Answer from the drawing. Dimensions are ordinates in mm from the lowest x, y and z of the part. A direction names the side the tool comes from. Coordinates: 2 decimals unless noted, no trailing zeros. Write each loop counter-clockwise with the first axis right and the second up, starting at its lowest first coordinate (ties: lowest second). Pieces come first, ordered by that corner, then holes.
(1) Given pin 1 (2 mm diameter, centred on y = 29.5, z = 9, fed in from +X); pin 2 (6 mm diameter, centred on x = 9, y = 26, fed in from -Z), each flat-ended and moving along its own axis, determine where each tip first touches the part or whether it passes through.
(2) Section D-D on y = 10 is taken. Write down the section's boundary in (x, z), then the cut area to 3 significant figures.
(3) Section A-A on z = 3.5 is taken. Write down the section's boundary in (x, y).
(4) The mould has two halves that part along Y. Classify the marked faces 1, 2 and 3: +Y half, -Y half, draft (parallel to the pull), parting line (faces both ways), or undercut.
(5) Find the intervals of material crossed by probe 1 along Y at (x, z) = (3.5, 9.5); probe 2 along Y at (x, z) = (6.5, 1); probe 3 along Z at (x, y) = (5.25, 4), in increasing order.
(6) Section C-C on x = 1 is taken. Write down the section's boundary in (y, z).
(7) Section B-B on y = 32 is taken. Write down the section's boundary in (x, z).
(8) Which of the six approach directions +Z, -Z, +X, -X, +Y, -Y give full straight-line access (tool end or side, diameter ignored) to the marked faces 4, 5 and 6?
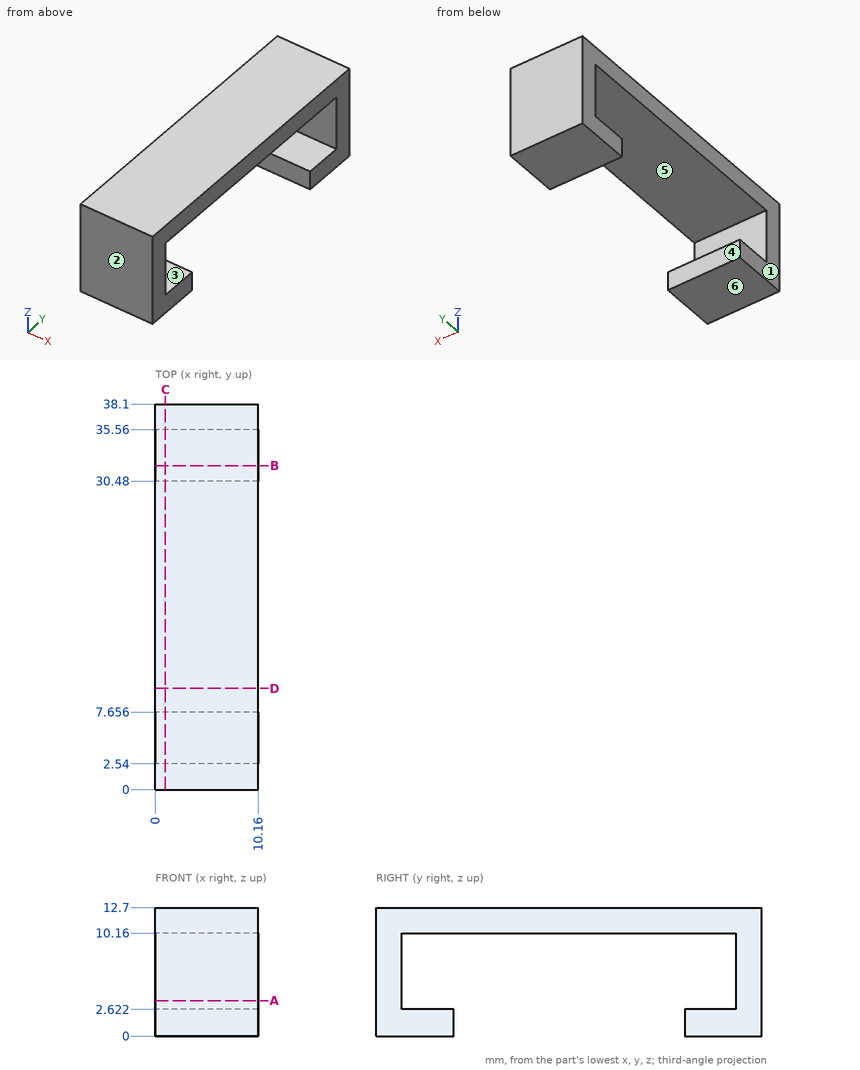
Response:
1. pin 1: passes through
1. pin 2: stops at z = 10.16
2. outline: (0, 10.16) - (10.16, 10.16) - (10.16, 12.7) - (0, 12.7) - close
2. area: 25.8 mm2
3. outline: (0, 0) - (10.16, 0) - (10.16, 2.54) - (0, 2.54) - close; (0, 35.56) - (10.16, 35.56) - (10.16, 38.1) - (0, 38.1) - close
4. face 1: draft
4. face 2: -Y half
4. face 3: undercut
5. probe 1: y = 0 to 2.54, 35.56 to 38.1
5. probe 2: y = 0 to 7.66, 30.48 to 38.1
5. probe 3: z = 0 to 2.62, 10.16 to 12.7
6. outline: (0, 0) - (7.66, 0) - (7.66, 2.62) - (2.54, 2.62) - (2.54, 10.16) - (35.56, 10.16) - (35.56, 2.62) - (30.48, 2.62) - (30.48, 0) - (38.1, 0) - (38.1, 12.7) - (0, 12.7) - close
7. outline: (0, 0) - (10.16, 0) - (10.16, 2.62) - (0, 2.62) - close; (0, 10.16) - (10.16, 10.16) - (10.16, 12.7) - (0, 12.7) - close
8. face 4: -Z, +X, -X
8. face 5: +X, -X
8. face 6: -Z, +X, -X, +Y, -Y
